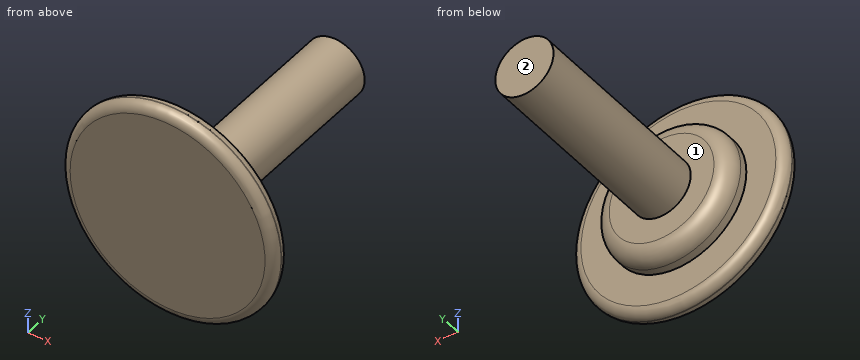
```python
from build123d import *

# Parameters (mm, degrees)
FILLET2_R = 1.524
FILLET3_R = 2.54


with BuildPart() as part:
    # Sketch1 → Base-Revolve (revolve)
    with BuildSketch(Plane.XY):
        Polygon((0, 0), (0, 38.1), (-4.7625, 38.1), (-4.7625, 6.985), (-11.1125, 6.985), (-11.1125, 3.175), (-17.4625, 3.175), (-17.4625, 0), align=None)
    revolve(axis=Axis((0, 0, 0), (0, 1, 0)))

    # Fillet2
    fillet2_edges = [part.edges().sort_by_distance(p)[0] for p in [
        (17.4625, 3.175, 0),
        (17.4625, 0, 0),
    ]]
    fillet(fillet2_edges, radius=FILLET2_R)

    # Fillet3
    fillet3_edges = [part.edges().sort_by_distance(p)[0] for p in [
        (11.1125, 6.985, 0),
    ]]
    fillet(fillet3_edges, radius=FILLET3_R)


solid = part.part
```
Part model, mm, in its own coordinate system. Face numbers are marked on the shaded views. A direction names the side the tool comes from. Round coordinates to 2 decimals unless told otherwise and drop trailing zeros. Write each loop counter-clockwise with the first axis right and the second up, starting at its lowest first coordinate (ties: lowest second). Pieces come first, ordered by that corner, then holes. Notation, with made-up numbers: (12, 69) -> (67, 69) arc R16 ccw to (67, 85) -> close; hole circle Ø9 at (85.25, 30). An arc over 180 degrees is marked (long way). Return JSON: item names as keys, results as strings. Group by question number.
Q1. Probe L1, parallel to Y at x = -11, z = -11 (3 decimals); L2, parallel to Z at x = 0, y = 34; L3, parallel to Y at x = 8.5, z = 4. List the from-to ranges inside material, lowest first. Write a range as [from, to].
Q2. Pin check, flat tips, straight feed: pin 1 (8 mm diameter, centred on x = 5, y = 24.5, fed in from -Z); pin 2 (5 mm diameter, centred on y = 22, z = -0.5, fed in from +X); pin 3 (6 mm diameter, centred on x = 2.5, z = 8, fed in from +Y) (3 decimals); pin 4 (16 mm diameter, centred on x = 6, z = 0, fed in from +Y). Stop position of each tip, or through.
Q3. Saw through at C-C on y = 32. Write the cut outline in (x, z) (1 decimal), plus the area to 3 significant figures.
Q4. Which spindle directions (+Z, -Z, +X, -X, +Y, -Y) get a long thin tool onto all of the face, cutting with end or side? Do the marked faces 1 and 2. Say none if no direction does.
Answer:
{
 "1": {"L1": "[0, 3.175]", "L2": "[-4.76, 4.76]", "L3": "[0, 6.85]"},
 "2": {"pin 1": "z = -4.66", "pin 2": "x = 4.76", "pin 3": "y = 6.985", "pin 4": "y = 38.1"},
 "3": {"outline": "circle Ø9.5 at (0, 0)", "area": "71.3 mm2"},
 "4": {"face 1": "+Y", "face 2": "+Z, -Z, +X, -X, +Y"}
}
